Input: part model. Units: mm. Frame: model coordinates. A direction names the side the tool comes from. Coordinates: 2 decimals unless noted, no trailing zeros. Write each loop counter-clockwise with the first axis right and the second up, starting at its lowest first coordinate (ties: lowest second). Pieces come first, ordered by that corner, then holes. Notation, with made-up numbers: (0, -28.5) -> (40, -28.5) arc R34 cw to (40, 8.5) -> close; hole circle Ø10 at (-25.5, 45). An arc over 180 degrees is marked (long way). One line per question, with ' | ' between items. Start each with the question number.
```python
from build123d import *

# Parameters (mm, degrees)
SKETCH2_R           = 1.15
RESISTOR_BODY_DEPTH = 6.4
LEAD1_PROFILE_R     = 0.3
SKETCH6_R           = 0.3
LEAD2_DEPTH         = 8.6


with BuildPart() as part:
    # Sketch2 → Resistor Body (new body)
    with BuildSketch(Plane.XY):
        Circle(SKETCH2_R)
    extrude(amount=RESISTOR_BODY_DEPTH)

    # Lead1: sweep along a path in Lead1 Path
    with BuildLine(Plane(origin=(0, 0, 0), x_dir=(-1, 0, 0), z_dir=(0, -1, 0))) as lead1_path:
        Line((0, -6.4), (0, -8.4))
        ThreePointArc((0, -8.4), (0.585786438, -9.814213562), (2, -10.4))
        Line((2, -10.4), (3, -10.4))
        ThreePointArc((3, -10.4), (4.414213562, -9.814213562), (5, -8.4))
        Line((5, -8.4), (5, 8.6))
    # Lead1 Profile → Lead1 (sweep)
    with BuildSketch(Plane(origin=(0, 0, 6.4), x_dir=(-1, 0, 0), z_dir=(0, 0, 1))):
        Circle(LEAD1_PROFILE_R)
    sweep(path=lead1_path.line)

    # Sketch6 → Lead2 (add)
    with BuildSketch(Plane(origin=(0, 0, 0), x_dir=(1, 0, 0), z_dir=(0, 0, -1))):
        Circle(SKETCH6_R)
    extrude(amount=LEAD2_DEPTH)


solid = part.part
```
1) First-contact query: P1, Ø0.7, axis at x = -0.5, y = -0.5, coming from the +Z side; P2, Ø3, axis at x = -4, z = 5.5, coming from the -Y side. Flat tips, straight axial feed; report the tip coordinate or a pass-through.
2) Section B-B, the plane y = 0. Return loops of the section in (x, z), then the cut area to 4 significant figures.
3) Section A-A, the plane z = -6.75. Return loops of the section in (x, y).
4) Ray query, line 1 (X direction, y = 0, z = -7); line 2 (Z direction, x = -0.25, y = -0.4); line 3 (X direction, y = -0.05, z = 9.25). Return the intervals inside material, ascending.
5) Section C-C, the plane z = 5.5. Return loops of the section in (x, y).
6) Access query for faces 1 (the face through (0, -0.5, 6.4)), 2 (the face through (0, -0.5, 0)). Directions: +Z, -Z, +X, -X, +Y, -Y. A direction counts if a zero-diameter tool reaches every point of the face in a straight line with its end or side. Return the directions, or none.
7) Section D-D, the plane y = -0.8. Return loops of the section in (x, z).
Answer block:
1) P1: stops at z = 10.19 | P2: stops at y = -0.3
2) outline: (-5.3, -8.6) -> (-4.7, -8.6) -> (-4.7, 8.4) arc R1.7 cw to (-3, 10.1) -> (-2, 10.1) arc R1.7 cw to (-0.3, 8.4) -> (-0.3, 6.4) -> (-1.15, 6.4) -> (-1.15, 0) -> (-0.3, 0) -> (-0.3, -8.6) -> (0.3, -8.6) -> (0.3, 0) -> (1.15, 0) -> (1.15, 6.4) -> (0.3, 6.4) -> (0.3, 8.4) arc R2.3 ccw to (-2, 10.7) -> (-3, 10.7) arc R2.3 ccw to (-5.3, 8.4) -> close | area: 35.65 mm2
3) outline: circle Ø0.6 at (-5, 0); circle Ø0.6 at (0, 0)
4) line 1: x = -5.3 to -4.7, -0.3 to 0.3 | line 2: z = 0 to 6.4 | line 3: x = -5.13 to -4.48, -0.52 to 0.13
5) outline: circle Ø0.6 at (-5, 0); circle Ø2.3 at (0, 0)
6) face 1: none | face 2: -Z
7) outline: (-0.83, 0) -> (0.83, 0) -> (0.83, 6.4) -> (-0.83, 6.4) -> close
